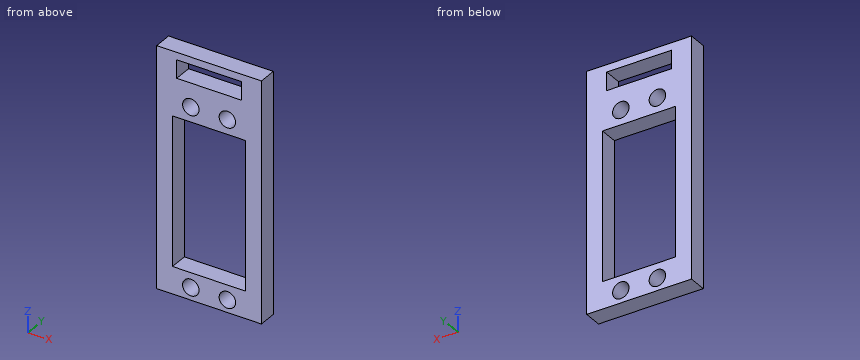
from build123d import *

# Parameters (mm, degrees)
SKETCH1_R           = 2.25
SKETCH1_W           = 20
SKETCH1_H           = 40.6
SKETCH1_W_2         = 17.696235852
SKETCH1_H_2         = 5
BOSS_EXTRUDE1_DEPTH = 5


with BuildPart() as part:
    # Sketch1 → Boss-Extrude1 (new body)
    with BuildSketch(Plane(origin=(0, 0, 0), x_dir=(1, 0, 0), z_dir=(0, 1, 0))):
        Polygon((-4.308878206, -48), (-4.308878206, 7.4), (24.308878206, 7.4), (24.308878206, -48), (24.308878206, -58.1), (-4.308878206, -58.1), align=None)
        with Locations(Location((5, 4, 0), (0, 0, 270))):
            Circle(SKETCH1_R, mode=Mode.SUBTRACT)
        with Locations(Location((15, 4, 0), (0, 0, 90))):
            Circle(SKETCH1_R, mode=Mode.SUBTRACT)
        with Locations(Location((5, -44.6, 0), (0, 0, 90))):
            Circle(SKETCH1_R, mode=Mode.SUBTRACT)
        with Locations(Location((15, -44.6, 0), (0, 0, 270))):
            Circle(SKETCH1_R, mode=Mode.SUBTRACT)
        with Locations((10, -20.3)):
            Rectangle(SKETCH1_W, SKETCH1_H, mode=Mode.SUBTRACT)
        with Locations((10, -53.6)):
            Rectangle(SKETCH1_W_2, SKETCH1_H_2, mode=Mode.SUBTRACT)
    extrude(amount=BOSS_EXTRUDE1_DEPTH)


solid = part.part
Work out the finished part from the listing and answer in its coordinate system (mm). Coordinates: 2 decimals unless noted, no trailing zeros. Loops run counter-clockwise (first coordinate to the right, second up) from the corner with the lowest first, then second, coordinate; pieces in that order, holes last. Notation, with made-up numbers: M 15.5,41.25 L 35.5,41.25 A20 ccw 35.5,76.25 Z; hole C 80,-1.5 d8. An arc over 180 degrees is marked long. Answer in a Markdown table with one row per item. Add a question column.
1. Consider L1, parallel to X at y = 3.85, z = 44.6; L2, parallel to Z at x = 11.75, y = 0.8; L3, parallel to X at y = 1.3, z = 22. Determine where each line is inside the solid, lowest interval first.
2. Find section A-A, the plane x = 8.75. Write down the section's boundary in (y, z), then the cut area to 3 significant figures.
3. A flat-ended cylindrical pin translates along its axis: P1, Ø3.5, axis at x = 5, z = -4, coming from the +Y side. Find the tip coordinate at first contact, or state that the pin passes through.
4. Find section B-B, the plane z = 6. Write down the section's boundary in (x, y).
5. Find section C-C, the plane z = 44.6. Write down the section's boundary in (x, y), then the cut area to 3 significant figures.
6. Find section D-D, the plane x = 5. Write down the section's boundary in (y, z), then the cut area to 3 significant figures.
Reported:
| question | item | result |
|---|---|---|
| 1 | L1 | x = -4.31 to 2.75, 7.25 to 12.75, 17.25 to 24.31 |
| 1 | L2 | z = -7.4 to 0, 40.6 to 51.1, 56.1 to 58.1 |
| 1 | L3 | x = -4.31 to 0, 20 to 24.31 |
| 2 | outline | M 0,-7.4 L 5,-7.4 L 5,0 L 0,0 Z; M 0,40.6 L 5,40.6 L 5,51.1 L 0,51.1 Z; M 0,56.1 L 5,56.1 L 5,58.1 L 0,58.1 Z |
| 2 | area | 99.5 mm^2 |
| 3 | P1 | passes through |
| 4 | outline | M -4.31,0 L 0,0 L 0,5 L -4.31,5 Z; M 20,0 L 24.31,0 L 24.31,5 L 20,5 Z |
| 5 | outline | M -4.31,0 L 2.75,0 L 2.75,5 L -4.31,5 Z; M 7.25,0 L 12.75,0 L 12.75,5 L 7.25,5 Z; M 17.25,0 L 24.31,0 L 24.31,5 L 17.25,5 Z |
| 5 | area | 98.1 mm^2 |
| 6 | outline | M 0,-7.4 L 5,-7.4 L 5,-6.25 L 0,-6.25 Z; M 0,-1.75 L 5,-1.75 L 5,0 L 0,0 Z; M 0,40.6 L 5,40.6 L 5,42.35 L 0,42.35 Z; M 0,46.85 L 5,46.85 L 5,51.1 L 0,51.1 Z; M 0,56.1 L 5,56.1 L 5,58.1 L 0,58.1 Z |
| 6 | area | 54.5 mm^2 |
